Can you work these out from the model? Positions are in its coordinate system, mm. A direction names the side the tool comes from. Coordinates: 2 decimals unless noted, no trailing zeros. Loops run counter-clockwise (first coordinate to the right, second up) from the corner with the lowest first, then second, coordinate; pieces in that order, holes last.
Autodesk Inventor part; units mm, degrees
ref_plane "YZ Plane" through (0, 0, 0) normal (1, 0, 0) x (0, 1, 0)
ref_plane "XZ Plane" through (0, 0, 0) normal (0, 1, 0) x (-1, 0, 0)
ref_plane "XY Plane" through (0, 0, 0) normal (0, 0, 1) x (1, 0, 0)
sketch "Sketch1" plane through (0, 0, 0) normal (0, 0, 1) x (1, 0, 0)
  line L0 (0, 116.9344) -> (0, -19.4891)
  line L1 (-17.2212, 0) -> (2.8702, 0)
  line L2 (0, 0) -> (0, 97.4453)
  line L3 (0, 0) -> (-13.6144, 0)
  line L4 (-13.6144, 0) -> (-14.351, 93.9546)
  line L5 (-14.351, 93.9546) -> (-13.2588, 93.9546)
  line L6 (-13.2588, 93.9546) -> (-12.5373, 1.9304)
  line L7 (-12.5373, 0) -> (-12.5373, 0.8382)
  line L8 (-12.5373, 0.8382) -> (0, 0.8382)
  line L9 (-12.5373, 1.9304) -> (0, 1.9304)
  line L10 (0, 1.9304) -> (0, 0.8382)
  dimension "d0" = 27.2288
  dimension "d1" = 28.702
  dimension "d2" = 93.9546
  dimension "d3" = 1.0922
  dimension "d5" = 0.8382
  dimension "d6" = 1.0922
  dimension "d9" = 26.5175
revolve "Revolution1" add sketch "Sketch1" angle 360 about axis through (0, 0, 0) along (0, 1, 0) contours L0 L8 L7 L1 L4 L5 L6 L9
fillet "Fillet1" radius 0.254 2 edges at (13.2588, 93.9546, 0) (14.351, 93.9546, 0)
Item 1: I'm going to push flat-ended pins straight in: P1, Ø3, axis at x = -9.5, z = -4.5, coming from the -Y side; P2, Ø1, axis at x = -11.5, y = 43, coming from the +Z side; P3, Ø1.5, axis at y = 84, z = -11, coming from the +X side. Where does each tip first touch, or does it pass through?
Results are:
P1: stops at y = 0.84
P2: stops at z = 8.58
P3: stops at x = 9.93
Item 2: We'd pull the mould along Z, two halves only. Please class faces 1 (the face through (-6.936, 48.459, 10.879)), 2 (the face through (3.032, 47.505, -13.654)), 3 (the face through (-9, 0, -9)): +Z half, -Z half, draft (parallel to the pull), parting line (faces both ways), or undercut.
Results are:
face 1: undercut
face 2: parting line
face 3: draft
Item 3: On a 3-axis mill with a long thin cutter (end or side, diameter ignored), from which of +Z, -Z, +X, -X, +Y, -Y can I reach the whole of each face in a straight line? I mean faces 4 (the face through (0, 1.93, 0)), 5 (the face through (0, 0.838, 0)). Say none if no direction works.
Results are:
face 4: +Y
face 5: -Y
Item 4: I need wall thicknesses on line 1 along Z through (x, y) = (0, 0.45); line 2 along Y through (x, z) = (-7, 0.5); line 3 along X through (y, z) = (11.5, -10.25). Which ranges of each line are inside material? Lowest first, please.
Results are:
line 1: z = -13.62 to -12.54, 12.54 to 13.62
line 2: y = 0.84 to 1.93
line 3: x = -9.1 to -7.35, 7.35 to 9.1
Item 5: Suppose I cut it at A-A, the plane y = 62. Please give me the cut outline in (x, z), plus the area to 3 significant figures.
Results are:
outline: circle Ø28.2 at (0, 0); hole circle Ø26.02 at (0, 0)
area: 93.0 mm2
Item 6: Suppose I cut it at B-B, the plane y = 8.5. Please give me the cut outline in (x, z).
Results are:
outline: circle Ø27.36 at (0, 0); hole circle Ø25.18 at (0, 0)
